```python
from build123d import *

# Parameters (mm, degrees)
SKETCH1_W            = 373.38
SKETCH1_H            = 449.58
BOSS_EXTRUDE1_DEPTH  = 1.5875
FILLET1_R            = 12.7
SKETCH2_R            = 3.175
CUT_EXTRUDE1_DEPTH   = 293.222142941
LPATTERN1_COUNT      = 4
LPATTERN1_PITCH      = 111.76
LPATTERN1_COUNT_DIR2 = 5
LPATTERN1_PITCH_DIR2 = 104.775
CUT_EXTRUDE2_DEPTH   = 303.544238838


with BuildPart() as part:
    # Sketch1 → Boss-Extrude1 (new, symmetric)
    with BuildSketch(Plane(origin=(0, 0, 0), x_dir=(1, 0, 0), z_dir=(0, 1, 0))):
        Rectangle(SKETCH1_W, SKETCH1_H)
    extrude(amount=BOSS_EXTRUDE1_DEPTH, both=True)

    # Fillet1
    fillet1_edges = [part.edges().sort_by_distance(p)[0] for p in [
        (186.69, 0, 224.79),
        (-186.69, 0, 224.79),
        (-186.69, 0, -224.79),
        (186.69, 0, -224.79),
    ]]
    fillet(fillet1_edges, radius=FILLET1_R)

    # Sketch2 → Cut-Extrude1 (cut, through all)
    with BuildSketch(Plane(origin=(0, 1.5875, 0), x_dir=(1, 0, 0), z_dir=(0, 1, 0))):
        with Locations(Location((-167.64, 209.55, 0), (0, 0, 270))):
            Circle(SKETCH2_R)
    cut_extrude1 = extrude(amount=-CUT_EXTRUDE1_DEPTH, mode=Mode.SUBTRACT)

    # LPattern1: Cut-Extrude1 4 × 5, 6 skipped
    with Locations(*[(i * LPATTERN1_PITCH, 0, j * LPATTERN1_PITCH_DIR2) for i in range(LPATTERN1_COUNT) for j in range(LPATTERN1_COUNT_DIR2) if (i, j) not in ((0, 0), (1, 1), (1, 2), (1, 3), (2, 1), (2, 2), (2, 3))]):
        add(cut_extrude1, mode=Mode.SUBTRACT)

    # Sketch3 → Cut-Extrude2 (cut, through all)
    with BuildSketch(Plane(origin=(13.560082756, 17.4625, -1.196765785), x_dir=(1, 0, 0), z_dir=(0, 1, 0))):
        with BuildLine():
            ThreePointArc((128.806917244, 113.692643266), (109.756917244, 109.293234215), (128.806917244, 104.893825163))
            Line((128.806917244, 104.893825163), (128.806917244, 113.692643266))
        make_face()
        with BuildLine():
            ThreePointArc((116.665717244, 150.635691209), (101.882917244, 147.393234215), (116.665717244, 144.15077722))
            Line((116.665717244, 144.15077722), (116.665717244, 150.635691209))
        make_face()
        with BuildLine():
            ThreePointArc((91.265717244, 150.635691209), (76.482917244, 147.393234215), (91.265717244, 144.15077722))
            Line((91.265717244, 144.15077722), (91.265717244, 150.635691209))
        make_face()
        with BuildLine():
            ThreePointArc((93.246917244, 113.692643266), (74.196917244, 109.293234215), (93.246917244, 104.893825163))
            Line((93.246917244, 104.893825163), (93.246917244, 113.692643266))
        make_face()
        with BuildLine():
            ThreePointArc((65.865717244, 150.635691209), (51.082917244, 147.393234215), (65.865717244, 144.15077722))
            Line((65.865717244, 144.15077722), (65.865717244, 150.635691209))
        make_face()
        with BuildLine():
            ThreePointArc((40.465717244, 150.635691209), (25.682917244, 147.393234215), (40.465717244, 144.15077722))
            Line((40.465717244, 144.15077722), (40.465717244, 150.635691209))
        make_face()
        with BuildLine():
            ThreePointArc((42.446917244, 113.692643266), (23.396917244, 109.293234215), (42.446917244, 104.893825163))
            Line((42.446917244, 104.893825163), (42.446917244, 113.692643266))
        make_face()
    extrude(amount=-CUT_EXTRUDE2_DEPTH, mode=Mode.SUBTRACT)


solid = part.part
```
Work out the finished part from the listing and answer in its coordinate system (mm). Coordinates: 2 decimals unless noted, no trailing zeros. Write each loop counter-clockwise with the first axis right and the second up, starting at its lowest first coordinate (ties: lowest second). Pieces come first, ordered by that corner, then holes.
Q1. This flat-tipped pin is pushed along its axis until it touches: pin 1 Ø4 at (x, z) = (167.64, 104.775) entering from -Y. Where does it stop, or does it pass through?
Q2. A cutting plane is placed at A-A, the plane x = 46.99. Give the vertices of the cut face in (y, z).
Q3. Find the intervals of material crossed by line 1 (Z direction, x = -167.64, y = -0.85) (3 decimals); line 2 (X direction, y = -0.9, z = 209.55) (3 decimals); line 3 (Z direction, x = 46.99, y = -0.25), in increasing order.
Q4. Determine the mould class of faces 1 (the face through (87.764, 0.022, -110.867)), 2 (the face through (-3, -1.588, -3)), 3 (the face through (-183.07, -0.02, -220.97)) for opening direction Z: released by +Z, released by -Z, zero draft, split by the parting line, or undercut.
Q5. A cutting plane is placed at B-B, the plane x = 135. Give the vertices of the cut face in (y, z), then the cut area to 3 significant figures.
Findings below:
1. pin 1: passes through
2. outline: (-1.59, -224.79) - (1.59, -224.79) - (1.59, -156.34) - (-1.59, -156.34) - close; (-1.59, -140.84) - (1.59, -140.84) - (1.59, -120.52) - (-1.59, -120.52) - close; (-1.59, -100.46) - (1.59, -100.46) - (1.59, 224.79) - (-1.59, 224.79) - close
3. line 1: z = -224.79 to -212.725, -206.375 to -107.95, -101.6 to -3.175, 3.175 to 101.6, 107.95 to 206.375, 212.725 to 224.79
3. line 2: x = -186.69 to -170.815, -164.465 to -59.055, -52.705 to 52.705, 59.055 to 164.465, 170.815 to 186.69
3. line 3: z = -224.79 to -156.34, -140.84 to -120.52, -100.46 to 224.79
4. face 1: undercut
4. face 2: zero draft
4. face 3: released by -Z
5. outline: (-1.59, -224.79) - (1.59, -224.79) - (1.59, -120.39) - (-1.59, -120.39) - close; (-1.59, -100.59) - (1.59, -100.59) - (1.59, 224.79) - (-1.59, 224.79) - close
5. area: 1,360 mm2
